Check sheet for the modelled part. Datum: model origin and axes. Units: mm. Face numbers are marked on the shaded views. A direction names the side the tool comes from. Coordinates: 2 decimals unless noted, no trailing zeros. Order: outer loops, then holes, each group sorted by start corner. A loop starts at its lowest first (then second) coordinate and runs counter-clockwise, first axis right, second up.
1. Cross-section at C-C (x = -19). Enter the section's corners in (y, z), then the cut area to 3 significant figures.
2. Gauge pin test, flat ends, axial feed: pin 1 Ø12 at (y, z) = (-26.5, 5) entering from -X; pin 2 Ø1.5 at (x, y) = (-59.5, -10) entering from +Z; pin 3 Ø5 at (y, z) = (-42.5, -26) entering from +X. Record the tip position at first contact, or that the pin passes through.
3. Draft check along X on the marked faces 6, 7 and 8. Enter one of: released by +X, released by -X, zero draft, split by the parting line, or undercut.
4. Set-up check for the marked faces 1, 2, 3, 4 and 5: record each of +Z, -Z, +X, -X, +Y, -Y from which the full face is reachable in a straight line by a thin tool's end or side.
5. Cross-section at A-A (z = -13). Enter the section's corners in (x, y), then the cut area to 3 significant figures.
6. Thickness scan on line 1 (X direction, y = -21, z = -26); line 2 (Y direction, x = 6.5, z = -5.5); line 3 (Y direction, x = 28, z = 7.5). Record the ranges inside material, lowest first.
7. Cross-section at B-B (y = -13.5). Enter the section's corners in (x, z).
8. Cross-section at D-D (z = 18). Enter the section's corners in (x, y).
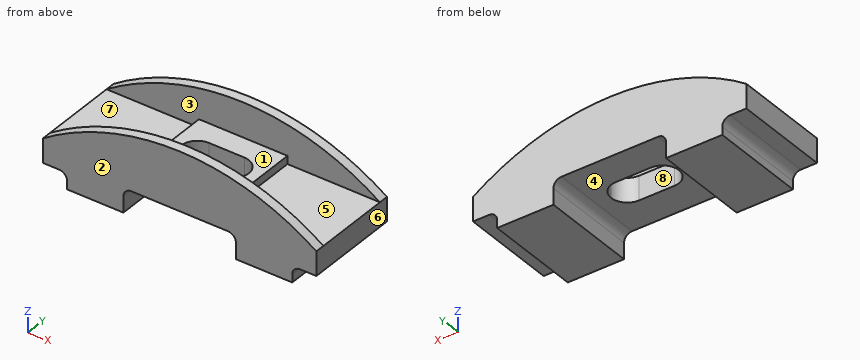
```python
from build123d import *

# Parameters (mm, degrees)
F1_DEPTH = 60
F3_DEPTH = 6
F5_DEPTH = 6
F7_DEPTH = 5
F9_DEPTH = 30.001


with BuildPart() as f1:
    # F0 (on Front) → F1 (new body)
    with BuildSketch(Plane.XZ):
        with BuildLine():
            Line((35, -30), (70, -30))
            Line((70, -30), (70, -25))
            ThreePointArc((70, -25), (71.4644660941, -21.4644660941), (75, -20))
            Line((75, -20), (85, -20))
            Line((85, -20), (85, -5))
            Line((85, -5), (-85, -5))
            Line((-85, -5), (-85, -20))
            Line((-85, -20), (-75, -20))
            ThreePointArc((-75, -20), (-71.4644660941, -21.4644660941), (-70, -25))
            Line((-70, -25), (-70, -30))
            Line((-70, -30), (-35, -30))
            Line((-35, -30), (-35, -20))
            ThreePointArc((-35, -20), (-33.5355339059, -16.4644660941), (-30, -15))
            Line((-30, -15), (30, -15))
            ThreePointArc((30, -15), (33.5355339059, -16.4644660941), (35, -20))
            Line((35, -20), (35, -30))
        make_face()
    extrude(amount=F1_DEPTH)

    # F2 (on face) → F3 (join)
    with BuildSketch(Plane(origin=(0, 0, 0), x_dir=(-1, 0, 0), z_dir=(0, 1, 0))):
        with BuildLine():
            Line((-85, -5), (85, -5))
            ThreePointArc((85, -5), (0, 21.4079290569), (-85, -5))
        make_face()
    extrude(amount=-F3_DEPTH)

    # F4 (on face) → F5 (join)
    with BuildSketch(Plane.XZ.offset(60)):
        with BuildLine():
            Line((-85, -5), (85, -5))
            ThreePointArc((85, -5), (0, 21.4079290569), (-85, -5))
        make_face()
    extrude(amount=-F5_DEPTH)

    # F6 (on face) → F7 (join)
    with BuildSketch(Plane.XY.offset(-5)):
        Polygon((27.5, -54), (27.5, -6), (0, -6), (-27.5, -6), (-27.5, -54), align=None)
    extrude(amount=F7_DEPTH)

    # F8 (on face) → F9 (cut, through all)
    with BuildSketch(Plane.XY):
        with BuildLine():
            Line((11, -20), (0, -20))
            Line((0, -20), (0, -30))
            Line((0, -30), (1, -30))
            ThreePointArc((1, -30), (3.9289321881, -22.9289321881), (11, -20))
        make_face()
        with BuildLine():
            Line((0, -30), (0, -20))
            Line((0, -20), (-11, -20))
            ThreePointArc((-11, -20), (-3.9289321881, -22.9289321881), (-1, -30))
            Line((-1, -30), (0, -30))
        make_face()
        with BuildLine():
            Line((1, -30), (0, -30))
            Line((0, -30), (0, -40))
            Line((0, -40), (11, -40))
            ThreePointArc((11, -40), (3.9289321881, -37.0710678119), (1, -30))
        make_face()
        with BuildLine():
            Line((0, -40), (0, -30))
            Line((0, -30), (-1, -30))
            ThreePointArc((-1, -30), (-3.9289321881, -37.0710678119), (-11, -40))
            Line((-11, -40), (0, -40))
        make_face()
        with BuildLine():
            Line((-11, -30), (-11, -20))
            ThreePointArc((-11, -20), (-21, -30), (-11, -40))
            Line((-11, -40), (-11, -30))
        make_face()
        with BuildLine():
            ThreePointArc((-1, -30), (-3.9289321881, -22.9289321881), (-11, -20))
            Line((-11, -20), (-11, -30))
            Line((-11, -30), (-1, -30))
        make_face()
        with BuildLine():
            Line((11, -30), (11, -20))
            ThreePointArc((11, -20), (3.9289321881, -22.9289321881), (1, -30))
            Line((1, -30), (11, -30))
        make_face()
        with BuildLine():
            ThreePointArc((21, -30), (18.0710678119, -22.9289321881), (11, -20))
            Line((11, -20), (11, -30))
            Line((11, -30), (11, -40))
            ThreePointArc((11, -40), (18.0710678119, -37.0710678119), (21, -30))
        make_face()
        with BuildLine():
            Line((11, -30), (1, -30))
            ThreePointArc((1, -30), (3.9289321881, -37.0710678119), (11, -40))
            Line((11, -40), (11, -30))
        make_face()
        with BuildLine():
            ThreePointArc((-11, -40), (-3.9289321881, -37.0710678119), (-1, -30))
            Line((-1, -30), (-11, -30))
            Line((-11, -30), (-11, -40))
        make_face()
    extrude(amount=-F9_DEPTH, mode=Mode.SUBTRACT)


solid = f1.part
```
Data:
1. outline: (-60, -15) - (-36, -15) - (-36, 0) - (-54, 0) - (-54, 20.2) - (-60, 20.2) - close; (-24, -15) - (0, -15) - (0, 20.2) - (-6, 20.2) - (-6, 0) - (-24, 0) - close
1. area: 962 mm2
2. pin 1: stops at x = -27.5
2. pin 2: stops at z = -5
2. pin 3: stops at x = 70.23
3. face 6: released by +X
3. face 7: zero draft
3. face 8: undercut
4. face 1: +Z, +X, -X
4. face 2: +Z, -Z, +X, -X, -Y
4. face 3: +Z
4. face 4: -Z, +Y, -Y
4. face 5: +Z, +X
5. outline: (-85, -60) - (85, -60) - (85, 0) - (-85, 0) - close; hole (-11, -40) - (11, -40) arc R10 ccw to (11, -20) - (-11, -20) arc R10 ccw to start
5. area: 9,450 mm2
6. line 1: x = -70 to -35, 35 to 70
6. line 2: y = -60 to -40, -20 to 0
6. line 3: y = -60 to -54, -6 to 0
7. outline: (-85, -20) - (-75, -20) arc R5 cw to (-70, -25) - (-70, -30) - (-35, -30) - (-35, -20) arc R5 cw to (-30, -15) - (30, -15) arc R5 cw to (35, -20) - (35, -30) - (70, -30) - (70, -25) arc R5 cw to (75, -20) - (85, -20) - (85, -5) - (27.5, -5) - (27.5, 0) - (-27.5, 0) - (-27.5, -5) - (-85, -5) - close
8. outline: (-31.79, -60) - (31.79, -60) - (31.79, -54) - (-31.79, -54) - close; (-31.79, -6) - (31.79, -6) - (31.79, 0) - (-31.79, 0) - close
